Design review of the part shown in the three views and the two pictorial views. Dimensions are in mm from the part's minimum x, y and z. A direction names the side the tool comes from. Round coordinates to 2 decimals unless told otherwise and drop trailing zeros. Write each loop counter-clockwise with the first axis right and the second up, starting at its lowest first coordinate (ties: lowest second). Pieces come first, ordered by that corner, then holes. Notation, with made-up numbers: (14.5, 35.5) -> (55.5, 35.5) arc R30 cw to (55.5, 62.5) -> close; hole circle Ø2 at (79.25, 24). An arc over 180 degrees is marked (long way). Answer as a JSON object with one key per item and string values. Group by question number.
1) Machinability: for the marked faces 1 and 2, which of the approach directions +Z, -Z, +X, -X, +Y, -Y give a long, thin tool a straight path to every point of the face, cutting with its end or side? Answer none if there is none.
2) To check wall thickness, follow probe 1 along X at (y, z) = (52.5, 396); probe 2 along Y at (x, z) = (66.5, 392). State the ranges of each line that lie inside material, in increasing order. Write a range as [from, to].
3) We need section C-C, the plane x = 589. Write out the cut boundary in (y, z).
4) We need section A-A, the plane y = 105. Write out the cut boundary in (x, z).
5) We need section B-B, the plane z = 53. Write out the cut boundary in (x, y).
6) Insertion check: pin 1 Ø8 at (x, z) = (310, 455) entering from -Y. The pin has a flat end and moves straight along its axis. Give the tip position at first contact, or say it passes through.
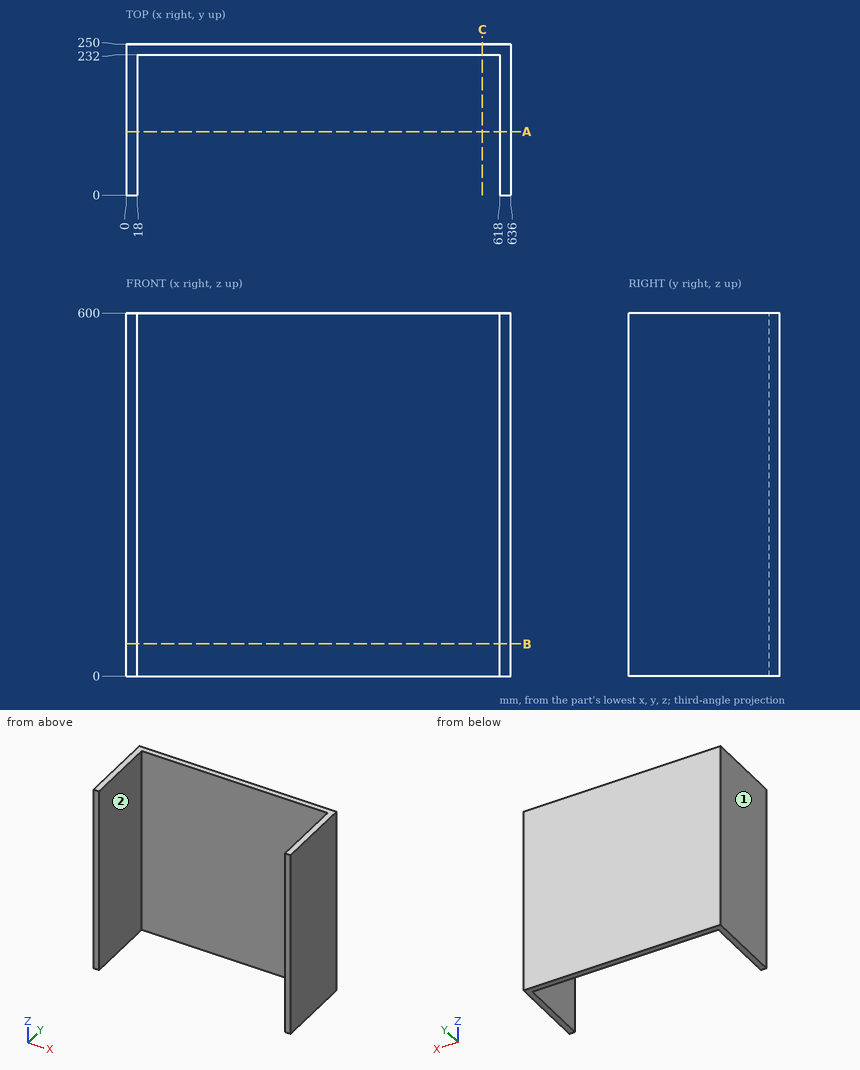
Here are the results:
{
 "1": {"face 1": "+Z, -Z, -X, +Y, -Y", "face 2": "+Z, -Z, -Y"},
 "2": {"probe 1": "x = [0, 18], [618, 636]", "probe 2": "y = [232, 250]"},
 "3": {"outline": "(232, 0) -> (250, 0) -> (250, 600) -> (232, 600) -> close"},
 "4": {"outline": "(0, 0) -> (18, 0) -> (18, 600) -> (0, 600) -> close; (618, 0) -> (636, 0) -> (636, 600) -> (618, 600) -> close"},
 "5": {"outline": "(0, 0) -> (18, 0) -> (18, 232) -> (618, 232) -> (618, 0) -> (636, 0) -> (636, 250) -> (0, 250) -> close"},
 "6": {"pin 1": "stops at y = 232"}
}
